Geometry: see drawing. Coordinates: mm, zero at the bounding-box minimum. Give positions to 0.01 mm unless a question says otherwise; leave off trailing zeros. Loops run counter-clockwise (first coordinate to the right, second up) from the corner with the lowest first, then second, coordinate; pieces in that order, holes last. Notation, with made-up numbers: M 3.5,67.25 L 61.5,67.25 A22 cw 61.5,102.25 Z; hole C -19.5,76 d10. An arc over 180 degrees is marked long. Answer in a Markdown table with one row per item.
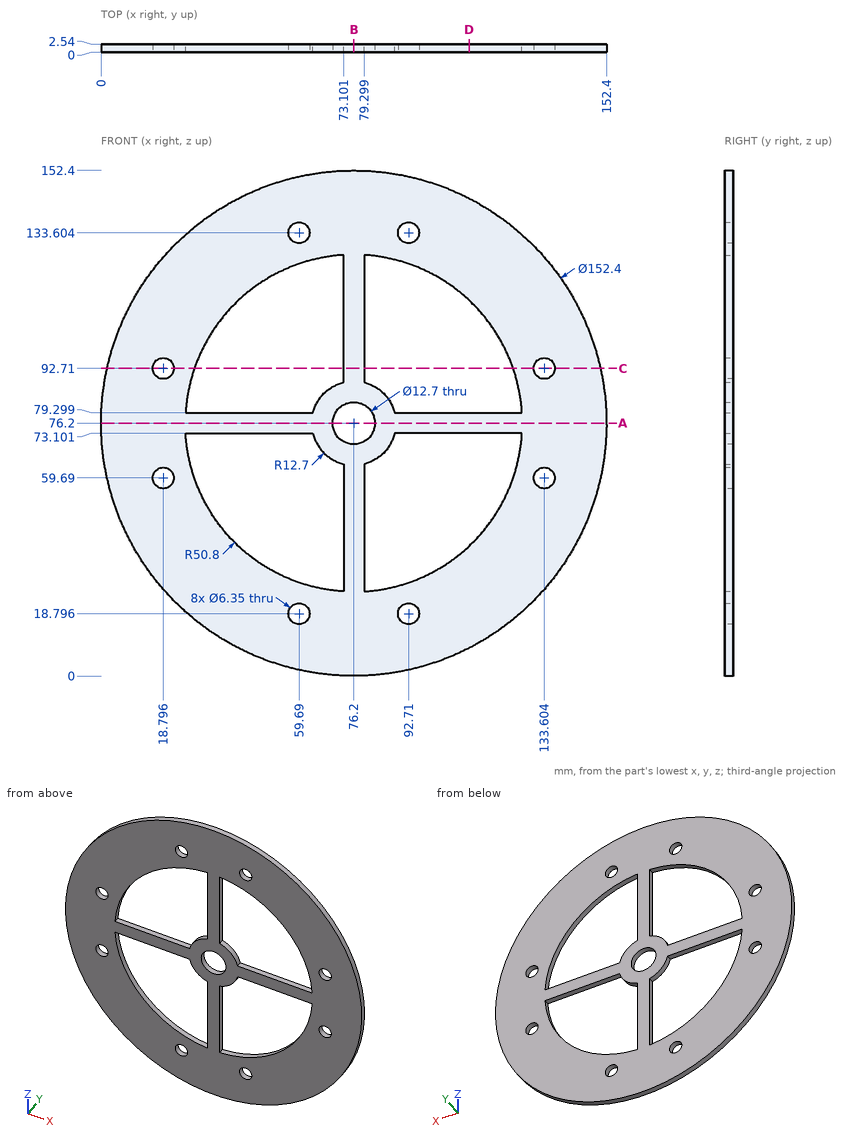
1) Pin query (flat end, axial travel): pin 1 Ø5.5 at (x, z) = (133.604, 92.71) entering from +Y; pin 2 Ø0.8 at (x, y) = (39, 1.5) entering from -Z (1 decimal); pin 3 Ø0.8 at (y, z) = (1, 112.5) entering from -X; pin 4 Ø1 at (x, y) = (123.5, 1) entering from +Z (1 decimal). Return the tip coordinate at first contact, or that it passes through.
Reply:
| item | result |
|---|---|
| pin 1 | passes through |
| pin 2 | stops at z = 9.5 |
| pin 3 | stops at x = 8.99 |
| pin 4 | stops at z = 136.3 |
2) Section B-B, the plane x = 76.2. Return loops of the section in (y, z).
Reply:
| item | result |
|---|---|
| outline | M 0,0 L 2.54,0 L 2.54,69.85 L 0,69.85 Z; M 0,82.55 L 2.54,82.55 L 2.54,152.4 L 0,152.4 Z |
3) Section A-A, the plane z = 76.2. Return loops of the section in (x, y), then the cut area to 3 significant figures.
Reply:
| item | result |
|---|---|
| outline | M 0,0 L 69.85,0 L 69.85,2.54 L 0,2.54 Z; M 82.55,0 L 152.4,0 L 152.4,2.54 L 82.55,2.54 Z |
| area | 355 mm² |
4) Section C-C, the plane z = 92.71. Return loops of the section in (x, y), then the cut area to 3 significant figures.
Reply:
| item | result |
|---|---|
| outline | M 1.81,0 L 15.62,0 L 15.62,2.54 L 1.81,2.54 Z; M 21.97,0 L 28.16,0 L 28.16,2.54 L 21.97,2.54 Z; M 73.1,0 L 79.3,0 L 79.3,2.54 L 73.1,2.54 Z; M 124.24,0 L 130.43,0 L 130.43,2.54 L 124.24,2.54 Z; M 136.78,0 L 150.59,0 L 150.59,2.54 L 136.78,2.54 Z |
| area | 117 mm² |
5) Section D-D, the plane x = 111. Return loops of the section in (y, z), then the cut area to 3 significant figures.
Reply:
| item | result |
|---|---|
| outline | M 0,8.41 L 2.54,8.41 L 2.54,39.19 L 0,39.19 Z; M 0,73.1 L 2.54,73.1 L 2.54,79.3 L 0,79.3 Z; M 0,113.21 L 2.54,113.21 L 2.54,143.99 L 0,143.99 Z |
| area | 172 mm² |
6) Material intervals for L1, parallel to Z at x = 109, y = 0.7; L2, parallel to X at y = 1.15, z = 59.69; L3, parallel to X at y = 2.3, z = 117.5 (1 decimal), sorted ascending.
Reply:
| item | result |
|---|---|
| L1 | z = 7.42 to 37.41, 73.1 to 79.3, 114.99 to 144.98 |
| L2 | x = 1.81 to 15.62, 21.97 to 28.16, 73.1 to 79.3, 124.24 to 130.43, 136.78 to 150.59 |
| L3 | x = 12.2 to 46.6, 73.1 to 79.3, 105.8 to 140.2 |
